Geometry check sheet. Reference: the model listing, model coordinates, mm. A direction names the side the tool comes from. Round coordinates to 2 decimals unless told otherwise and drop trailing zeros. Write each loop counter-clockwise with the first axis right and the second up, starting at its lowest first coordinate (ties: lowest second). Pieces come first, ordered by that corner, then holes. Notation, with made-up numbers: (50.25, 83) -> (57.25, 83) arc R19 ccw to (57.25, 89) -> close; hole circle Ø8 at (38.5, -11.75). An arc over 180 degrees is marked (long way). Return JSON: item names as keys, results as strings. Group by question number.
from build123d import *

# Parameters (mm, degrees)
SKETCH2_W           = 27
SKETCH2_H           = 27
BOSS_EXTRUDE1_DEPTH = 8
SKETCH5_R           = 0.6
CUT_EXTRUDE2_DEPTH  = 8
SKETCH2_6_W         = 27
SKETCH2_6_H         = 27
SKETCH2_6_W_2       = 20
SKETCH2_6_H_2       = 20
BOSS_EXTRUDE2_DEPTH = 43


with BuildPart() as part:
    # Sketch2 → Boss-Extrude1 (new body)
    with BuildSketch(Plane.XY.offset(43)):
        Rectangle(SKETCH2_W, SKETCH2_H)
    extrude(amount=BOSS_EXTRUDE1_DEPTH)

    # Sketch5 → Cut-Extrude2 (cut)
    with BuildSketch(Plane.XY.offset(43)):
        with Locations((-8.23, 8.23)):
            Circle(SKETCH5_R)
        with Locations((-5.88, 8.23)):
            Circle(SKETCH5_R)
        with Locations((-3.53, 8.23)):
            Circle(SKETCH5_R)
        with Locations((-1.18, 8.23)):
            Circle(SKETCH5_R)
        with Locations((1.17, 8.23)):
            Circle(SKETCH5_R)
        with Locations((3.52, 8.23)):
            Circle(SKETCH5_R)
        with Locations((5.87, 8.23)):
            Circle(SKETCH5_R)
        with Locations((8.22, 8.23)):
            Circle(SKETCH5_R)
        with Locations((-5.88, 5.88)):
            Circle(SKETCH5_R)
        with Locations((-3.53, 5.88)):
            Circle(SKETCH5_R)
        with Locations((-1.18, 5.88)):
            Circle(SKETCH5_R)
        with Locations((1.17, 5.88)):
            Circle(SKETCH5_R)
        with Locations((3.52, 5.88)):
            Circle(SKETCH5_R)
        with Locations((5.87, 5.88)):
            Circle(SKETCH5_R)
        with Locations((8.22, 5.88)):
            Circle(SKETCH5_R)
        with Locations((-5.88, 3.53)):
            Circle(SKETCH5_R)
        with Locations((-3.53, 3.53)):
            Circle(SKETCH5_R)
        with Locations((-1.18, 3.53)):
            Circle(SKETCH5_R)
        with Locations((1.17, 3.53)):
            Circle(SKETCH5_R)
        with Locations((3.52, 3.53)):
            Circle(SKETCH5_R)
        with Locations((5.87, 3.53)):
            Circle(SKETCH5_R)
        with Locations((8.22, 3.53)):
            Circle(SKETCH5_R)
        with Locations((-5.88, 1.18)):
            Circle(SKETCH5_R)
        with Locations((-3.53, 1.18)):
            Circle(SKETCH5_R)
        with Locations((-1.18, 1.18)):
            Circle(SKETCH5_R)
        with Locations((1.17, 1.18)):
            Circle(SKETCH5_R)
        with Locations((3.52, 1.18)):
            Circle(SKETCH5_R)
        with Locations((5.87, 1.18)):
            Circle(SKETCH5_R)
        with Locations((8.22, 1.18)):
            Circle(SKETCH5_R)
        with Locations((-5.88, -1.17)):
            Circle(SKETCH5_R)
        with Locations((-3.53, -1.17)):
            Circle(SKETCH5_R)
        with Locations((-1.18, -1.17)):
            Circle(SKETCH5_R)
        with Locations((1.17, -1.17)):
            Circle(SKETCH5_R)
        with Locations((3.52, -1.17)):
            Circle(SKETCH5_R)
        with Locations((5.87, -1.17)):
            Circle(SKETCH5_R)
        with Locations((8.22, -1.17)):
            Circle(SKETCH5_R)
        with Locations((-5.88, -3.52)):
            Circle(SKETCH5_R)
        with Locations((-3.53, -3.52)):
            Circle(SKETCH5_R)
        with Locations((-1.18, -3.52)):
            Circle(SKETCH5_R)
        with Locations((1.17, -3.52)):
            Circle(SKETCH5_R)
        with Locations((3.52, -3.52)):
            Circle(SKETCH5_R)
        with Locations((5.87, -3.52)):
            Circle(SKETCH5_R)
        with Locations((8.22, -3.52)):
            Circle(SKETCH5_R)
        with Locations((-5.88, -5.87)):
            Circle(SKETCH5_R)
        with Locations((-3.53, -5.87)):
            Circle(SKETCH5_R)
        with Locations((-1.18, -5.87)):
            Circle(SKETCH5_R)
        with Locations((1.17, -5.87)):
            Circle(SKETCH5_R)
        with Locations((3.52, -5.87)):
            Circle(SKETCH5_R)
        with Locations((5.87, -5.87)):
            Circle(SKETCH5_R)
        with Locations((8.22, -5.87)):
            Circle(SKETCH5_R)
        with Locations((-5.88, -8.22)):
            Circle(SKETCH5_R)
        with Locations((-3.53, -8.22)):
            Circle(SKETCH5_R)
        with Locations((-1.18, -8.22)):
            Circle(SKETCH5_R)
        with Locations((1.17, -8.22)):
            Circle(SKETCH5_R)
        with Locations((3.52, -8.22)):
            Circle(SKETCH5_R)
        with Locations((5.87, -8.22)):
            Circle(SKETCH5_R)
        with Locations((8.22, -8.22)):
            Circle(SKETCH5_R)
        with Locations((-8.23, 5.88)):
            Circle(SKETCH5_R)
        with Locations((-8.23, 3.53)):
            Circle(SKETCH5_R)
        with Locations((-8.23, 1.18)):
            Circle(SKETCH5_R)
        with Locations((-8.23, -1.17)):
            Circle(SKETCH5_R)
        with Locations((-8.23, -3.52)):
            Circle(SKETCH5_R)
        with Locations((-8.23, -5.87)):
            Circle(SKETCH5_R)
        with Locations((-8.23, -8.22)):
            Circle(SKETCH5_R)
    extrude(amount=CUT_EXTRUDE2_DEPTH, mode=Mode.SUBTRACT)

    # Sketch2<6> → Boss-Extrude2 (add)
    with BuildSketch(Plane.XY.offset(43)):
        Rectangle(SKETCH2_6_W, SKETCH2_6_H)
        Rectangle(SKETCH2_6_W_2, SKETCH2_6_H_2, mode=Mode.SUBTRACT)
    extrude(amount=-BOSS_EXTRUDE2_DEPTH)


solid = part.part
1) Tool access check on faces 1 (the face through (-4.006, -1.535, 46.944)), 2 (the face through (0, 0, 43)). Record the directions out of +Z, -Z, +X, -X, +Y, -Y that give a thin tool (end or side, any length) a straight path to the whole face; none if there is none.
2) Material ranges on probe 1 along X at (y, z) = (4, 12); probe 2 along Z at (x, y) = (3, 0), recorded low to high. Write a range as [from, to].
3) Sectioned sample at A-A on y = -8.22. State how many separate pieces and enclosed holes the cut face has, and give its area (3 significant figures).
4) Mould release check, pull along Y, two halves, no side actions. Record for faces 3 (the face through (-3.608, -7.625, 46.944)), 4 (the face through (0, 13.5, 26)): +Y half, -Y half, draft (parallel to the pull), parting line (faces both ways), or undercut.
5) Sectioned sample at B-B on z = 12. Enter the section's corners in (x, y).
6) Go/stop test with a flat-tipped pin: P1, Ø1.9, axis at x = -3.53, y = -1.17, coming from the -Z side. Record where the tip stops, or that it passes through.
Evaluation:
{
 "1": {"face 1": "+Z, -Z", "face 2": "-Z"},
 "2": {"probe 1": "x = [-13.5, -10], [10, 13.5]", "probe 2": "z = [43, 51]"},
 "3": {"separate pieces": "9", "enclosed holes": "0", "area": "440 mm2"},
 "4": {"face 3": "undercut", "face 4": "+Y half"},
 "5": {"outline": "(-13.5, -13.5) -> (13.5, -13.5) -> (13.5, 13.5) -> (-13.5, 13.5) -> close; hole (-10, -10) -> (10, -10) -> (10, 10) -> (-10, 10) -> close"},
 "6": {"P1": "stops at z = 43"}
}
